Geometry check sheet. Reference: the model listing, model coordinates, mm. A direction names the side the tool comes from. Coordinates: 2 decimals unless noted, no trailing zeros. Order: outer loops, then holes, each group sorted by start corner. A loop starts at its lowest first (then second) coordinate and runs counter-clockwise, first axis right, second up. Notation, with made-up numbers: (-13.5, 28) - (20.5, 28) arc R19 ccw to (20.5, 35) - close; hole circle Ø9 at (-32.5, -33.75). An arc over 180 degrees is marked (long way). Put each result on its own line as item: value.
from build123d import *

# Parameters (mm, degrees)
SKETCH_2_W               = 10
SKETCH_2_H               = 10
EXTRUDE_1_DEPTH          = 25
SKETCH_3_R               = 1.5
CUT_EXTRUDE_1_DEPTH      = 28.386127875
CUT_EXTRUDE_2_DEPTH      = 51.497524692
CUT_EXTRUDE_2_DEPTH_BACK = 51.497524692
SKETCH_4_W               = 6
SKETCH_4_H               = 6


with BuildPart() as part:
    # 草图2 → 凸台-拉伸1 (new, symmetric)
    with BuildSketch(Plane.XY):
        Rectangle(SKETCH_2_W, SKETCH_2_H)
    extrude(amount=EXTRUDE_1_DEPTH, both=True)

    # 草图3 → 切除-拉伸1 (cut, symmetric)
    with BuildSketch(Plane(origin=(0, 5, 0), x_dir=(1, 0, 0), z_dir=(0, 1, 0))):
        with Locations(Location((0, 17, 0), (0, 0, 270))):
            Circle(SKETCH_3_R)
    cut_extrude_1 = extrude(amount=CUT_EXTRUDE_1_DEPTH, both=True, mode=Mode.SUBTRACT)

    # 镜向1: 切除-拉伸1 across plane
    add(cut_extrude_1.mirror(Plane.XY), mode=Mode.SUBTRACT)

    # 草图4 → 切除-拉伸2 (cut, two sides: drawn at the far end of the back side and taken through both)
    with BuildSketch(Plane.XY.offset(25).offset(-CUT_EXTRUDE_2_DEPTH_BACK)):
        Rectangle(SKETCH_4_W, SKETCH_4_H)
    extrude(amount=CUT_EXTRUDE_2_DEPTH + CUT_EXTRUDE_2_DEPTH_BACK, mode=Mode.SUBTRACT)


solid = part.part
Q1. Draft check along Z on faces 1 (the flat face through (0, 3, 0)), 2 (the cylindrical face through (0.07, -3.99, -18.5)), 3 (the flat face through (-0.1, 3.4, -25)). Enter one of: pulls with the +Z half, pulls with the -Z half, needs draft (parallel to the pull), parting line crosses it, or undercut.
Answer block:
face 1: needs draft
face 2: undercut
face 3: pulls with the -Z half
Q2. Access from +Z, -Z, +X, -X, +Y, -Y to the whole of each face (thin tool, end or side, straight path). Record for faces 4 (the flat face through (0, 5, 0)), 5 (the flat face through (-3, 0, 0)).
Answer block:
face 4: +Z, -Z, +X, -X, +Y
face 5: +Z, -Z
Q3. Section check A-A on z = -13. Record the boundary of the cut face in (x, y).
Answer block:
outline: (-5, -5) - (5, -5) - (5, 5) - (-5, 5) - close; hole (-3, -3) - (3, -3) - (3, 3) - (-3, 3) - close
Q4. Thickness scan on L1, parallel to X at y = -2.75, z = 19; L2, parallel to X at y = -3.95, z = 17. Record the ranges inside material, lowest first. Write a range as [from, to].
Answer block:
L1: x = [-5, -3], [3, 5]
L2: x = [-5, -1.5], [1.5, 5]
Q5. Section check D-D on z = 17. Record the boundary of the cut face in (x, y).
Answer block:
outline: (-5, -5) - (-1.5, -5) - (-1.5, -3) - (-3, -3) - (-3, 3) - (-1.5, 3) - (-1.5, 5) - (-5, 5) - close; (1.5, -5) - (5, -5) - (5, 5) - (1.5, 5) - (1.5, 3) - (3, 3) - (3, -3) - (1.5, -3) - close
Q6. Section check B-B on y = -2. Record the boundary of the cut face in (x, z).
Answer block:
outline: (-5, -25) - (-3, -25) - (-3, 25) - (-5, 25) - close; (3, -25) - (5, -25) - (5, 25) - (3, 25) - close
